```python
from build123d import *

# Parameters (mm, degrees)
EXTRUDE_START   = -492.5
EXTRUDE_1_DEPTH = 492.5


with BuildPart() as part:
    # Эскиз1 → Бобышка-Вытянуть1 (new body)
    with BuildSketch(Plane.XY.offset(EXTRUDE_START)):
        with BuildLine():
            Line((-22, 50), (22, 50))
            ThreePointArc((22, 50), (24.121320344, 49.121320344), (25, 47))
            Line((25, 47), (25, 3))
            ThreePointArc((25, 3), (24.121320344, 0.878679656), (22, 0))
            Line((22, 0), (-22, 0))
            ThreePointArc((-22, 0), (-24.121320344, 0.878679656), (-25, 3))
            Line((-25, 3), (-25, 47))
            ThreePointArc((-25, 47), (-24.121320344, 49.121320344), (-22, 50))
        make_face()
        with BuildLine():
            Line((-20, 47), (20, 47))
            ThreePointArc((20, 47), (21.414213562, 46.414213562), (22, 45))
            Line((22, 45), (22, 5))
            ThreePointArc((22, 5), (21.414213562, 3.585786438), (20, 3))
            Line((20, 3), (-20, 3))
            ThreePointArc((-20, 3), (-21.414213562, 3.585786438), (-22, 5))
            Line((-22, 5), (-22, 45))
            ThreePointArc((-22, 45), (-21.414213562, 46.414213562), (-20, 47))
        make_face(mode=Mode.SUBTRACT)
    extrude(amount=EXTRUDE_1_DEPTH)


solid = part.part
```
Geometry check sheet. Reference: the model listing, model coordinates, mm. A direction names the side the tool comes from. Round coordinates to 2 decimals unless told otherwise and drop trailing zeros. Write each loop counter-clockwise with the first axis right and the second up, starting at its lowest first coordinate (ties: lowest second). Pieces come first, ordered by that corner, then holes. Notation, with made-up numbers: (12, 10) - (28, 10) arc R25 cw to (28, 29) - close; hole circle Ø6 at (28, -35). An arc over 180 degrees is marked (long way). Write each question's results on one line, items separated by ' | '.
(1) Draft check along X on faces 1 (the face through (0, 50, -250)), 2 (the face through (-25, 25, -250)), 3 (the face through (0, 3, -250)), 4 (the face through (-22, 25, -250)). Enter one of: pulls with the +X half, pulls with the -X half, needs draft (parallel to the pull), parting line crosses it, or undercut.
Computed:
face 1: needs draft | face 2: pulls with the -X half | face 3: undercut | face 4: undercut
(2) Thickness scan on probe 1 along Y at (x, z) = (14.5, -92); probe 2 along X at (y, z) = (29, -154.5); probe 3 along X at (y, z) = (46, -240.5). Record the ranges inside material, lowest first. Write a range as from..to.
Computed:
probe 1: y = 0..3, 47..50 | probe 2: x = -25..-22, 22..25 | probe 3: x = -25..-21.73, 21.73..25
(3) Sectioned sample at A-A, the plane x = 4.5. Enter the section's corners in (y, z), plus the area to 4 significant figures.
Computed:
outline: (0, -492.5) - (3, -492.5) - (3, 0) - (0, 0) - close; (47, -492.5) - (50, -492.5) - (50, 0) - (47, 0) - close | area: 2,955 mm^2
(4) Sectioned sample at C-C, the plane z = -87.5. Enter the section's corners in (x, y).
Computed:
outline: (-25, 3) arc R3 ccw to (-22, 0) - (22, 0) arc R3 ccw to (25, 3) - (25, 47) arc R3 ccw to (22, 50) - (-22, 50) arc R3 ccw to (-25, 47) - close; hole (-22, 5) arc R2 ccw to (-20, 3) - (20, 3) arc R2 ccw to (22, 5) - (22, 45) arc R2 ccw to (20, 47) - (-20, 47) arc R2 ccw to (-22, 45) - close
(5) Sectioned sample at B-B, the plane y = 17. Enter the section's corners in (x, z), plus the area to 4 significant figures.
Computed:
outline: (-25, -492.5) - (-22, -492.5) - (-22, 0) - (-25, 0) - close; (22, -492.5) - (25, -492.5) - (25, 0) - (22, 0) - close | area: 2,955 mm^2
(6) Set-up check for faces 5 (the face through (0, 0, -250)), 6 (the face through (22, 25, -250)): record each of +Z, -Z, +X, -X, +Y, -Y from which the full face is reachable in a straight line by a thin tool's end or side.
Computed:
face 5: +Z, -Z, +X, -X, -Y | face 6: +Z, -Z
